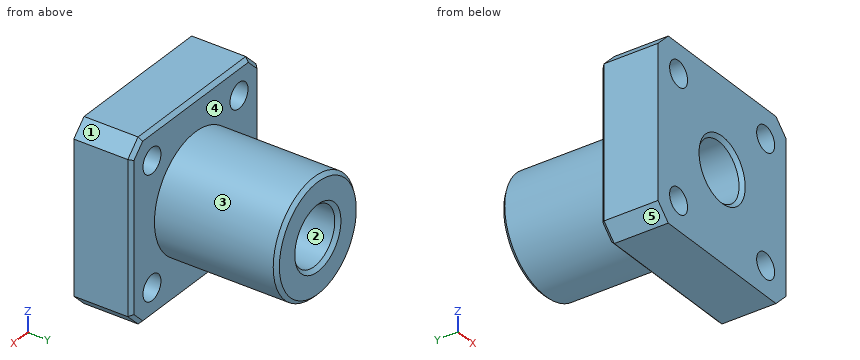
from build123d import *

# Parameters (mm, degrees)
ESQUISSE1_W      = 25
ESQUISSE1_H      = 25
ESQUISSE1_R      = 1.75
EXTRUSION1_DEPTH = 8
ESQUISSE2_R      = 8
EXTRUSION2_DEPTH = 17
CHANFREIN1_SIZE  = 2
EXTRUSION3_REACH = 27
ESQUISSE3_R      = 4
CHANFREIN2_SIZE  = 0.5


with BuildPart() as part:
    # Esquisse1 → Extrusion1 (new body)
    with BuildSketch(Plane(origin=(0, 0, 0), x_dir=(1, 0, 0), z_dir=(0, 1, 0))):
        with Locations((12.5, 12.5)):
            Rectangle(ESQUISSE1_W, ESQUISSE1_H)
        with Locations((4.014718626, 20.985281374)):
            Circle(ESQUISSE1_R, mode=Mode.SUBTRACT)
        with Locations((20.985281374, 20.985281374)):
            Circle(ESQUISSE1_R, mode=Mode.SUBTRACT)
        with Locations((20.985281374, 4.014718626)):
            Circle(ESQUISSE1_R, mode=Mode.SUBTRACT)
        with Locations((4.014718626, 4.014718626)):
            Circle(ESQUISSE1_R, mode=Mode.SUBTRACT)
    extrude(amount=EXTRUSION1_DEPTH)

    # Esquisse2 → Extrusion2 (add)
    with BuildSketch(Plane(origin=(0, 8, 0), x_dir=(1, 0, 0), z_dir=(0, 1, 0))):
        with Locations((12.5, 12.5)):
            Circle(ESQUISSE2_R)
    extrude(amount=EXTRUSION2_DEPTH)

    # Chanfrein1
    chanfrein1_edges = [part.edges().sort_by_distance(p)[0] for p in [
        (0, 4, -25),
        (25, 4, -25),
        (25, 4, 0),
        (0, 4, 0),
    ]]
    chamfer(chanfrein1_edges, length=CHANFREIN1_SIZE)

    # Esquisse3 → Extrusion3 (cut, up to next)
    with BuildSketch(Plane(origin=(0, 25, 0), x_dir=(1, 0, 0), z_dir=(0, 1, 0)), mode=Mode.PRIVATE) as extrusion3_sk1:
        with Locations((12.5, 12.5)):
            Circle(ESQUISSE3_R)
    extrusion3_tool1 = extrude(extrusion3_sk1.sketch, amount=-EXTRUSION3_REACH, mode=Mode.PRIVATE) & part.part
    add(extrusion3_tool1.solids().sort_by_distance((12.5, 25, -12.5))[0], mode=Mode.SUBTRACT)

    # Chanfrein2
    chanfrein2_edges = [part.edges().sort_by_distance(p)[0] for p in [
        (4.5, 25, -12.5),
        (0, 8, -12.5),
        (12.5, 8, -25),
        (12.5, 8, 0),
        (25, 8, -12.5),
        (1, 8, -1),
        (24, 8, -1),
        (24, 8, -24),
        (1, 8, -24),
        (8.5, 0, -12.5),
        (8.5, 25, -12.5),
    ]]
    chamfer(chanfrein2_edges, length=CHANFREIN2_SIZE)


solid = part.part
Work out the finished part from the listing and answer in its coordinate system (mm). Face numbers are marked on the shaded views. A direction names the side the tool comes from. Round coordinates to 2 decimals unless told otherwise and drop trailing zeros. Write each loop counter-clockwise with the first axis right and the second up, starting at its lowest first coordinate (ties: lowest second). Pieces come first, ordered by that corner, then holes.
1) Given pin 1 Ø5 at (x, y) = (13, 14.5) entering from +Z; pin 2 Ø1.5 at (y, z) = (19, -13) entering from -X; pin 3 Ø1 at (x, y) = (14.5, 18.5) entering from +Z, each flat-ended and moving along its own axis, determine where each tip first touches the part or whether it passes through.
2) Straight lines are drawn through the part: line 1 (X direction, y = 17.75, z = -12.5); line 2 (Z direction, x = 12.5, y = 19.25); line 3 (Z direction, x = 4.5, y = 7.25). For each, find the intervals that lie inside material, in ascending order.
3) A cutting plane is placed at C-C (y = 5.5). Give the vertices of the cut face in (x, z).
4) The mould has two halves that part along X. Classify the marked faces 1, 2 and 3: pulls with the +X half, pulls with the -X half, needs draft (parallel to the pull), parting line crosses it, or undercut.
5) A tool of negligible diameter and unlimited length cuts with its end or side. For the marked faces 4 and 5, from which of +Z, -Z, +X, -X, +Y, -Y can it reach the whole face along a straight path? Write none if from no direction.
6) A cutting plane is placed at B-B (z = -12.5). Give the vertices of the cut face in (x, y).
7) A cutting plane is placed at D-D (z = -3). Give the vertices of the cut face in (x, y), plus the area to 3 significant figures.
8) A cutting plane is placed at A-A (x = 12.5). Give the vertices of the cut face in (y, z), plus the area to 3 significant figures.
Completed:
1. pin 1: stops at z = -4.5
1. pin 2: stops at x = 4.5
1. pin 3: stops at z = -4.64
2. line 1: x = 4.5 to 8.5, 16.5 to 20.5
2. line 2: z = -20.5 to -16.5, -8.5 to -4.5
2. line 3: z = -25 to -22.67, -19.3 to -5.7, -2.33 to 0
3. outline: (0, -23) - (2, -25) - (23, -25) - (25, -23) - (25, -2) - (23, 0) - (2, 0) - (0, -2) - close; hole circle Ø3.5 at (4.01, -20.99); hole circle Ø3.5 at (4.01, -4.01); hole circle Ø8 at (12.5, -12.5); hole circle Ø3.5 at (20.99, -20.99); hole circle Ø3.5 at (20.99, -4.01)
4. face 1: pulls with the +X half
4. face 2: undercut
4. face 3: parting line crosses it
5. face 4: +Y
5. face 5: -Z, -X, +Y, -Y
6. outline: (0, 0) - (8, 0) - (8.5, 0.5) - (8.5, 24.5) - (8, 25) - (5, 25) - (4.5, 24.5) - (4.5, 8) - (0.5, 8) - (0, 7.5) - close; (16.5, 0.5) - (17, 0) - (25, 0) - (25, 7.5) - (24.5, 8) - (20.5, 8) - (20.5, 24.5) - (20, 25) - (17, 25) - (16.5, 24.5) - close
7. outline: (0, 0) - (2.59, 0) - (2.59, 8) - (0.5, 8) - (0, 7.5) - close; (5.44, 0) - (19.56, 0) - (19.56, 8) - (5.44, 8) - close; (22.41, 0) - (25, 0) - (25, 7.5) - (24.5, 8) - (22.41, 8) - close
7. area: 154 mm2
8. outline: (0, -25) - (7.5, -25) - (8, -24.5) - (8, -20.5) - (24.5, -20.5) - (25, -20) - (25, -17) - (24.5, -16.5) - (0.5, -16.5) - (0, -17) - close; (0, -8) - (0.5, -8.5) - (24.5, -8.5) - (25, -8) - (25, -5) - (24.5, -4.5) - (8, -4.5) - (8, -0.5) - (7.5, 0) - (0, 0) - close
8. area: 271 mm2
